```python
from build123d import *

# Parameters (mm, degrees)
F0_R     = 7.9375
F1_DEPTH = 14.2748
F2_R     = 1.1303
F3_DEPTH = 12.701


with BuildPart() as f1:
    # F0 (on Top) → F1 (new body)
    with BuildSketch(Plane.XY):
        Polygon((57.15, -9.525), (57.15, 9.525), (28.109774, 9.525), (28.109774, 3.175), (-28.109774, 3.175), (-28.109774, 9.525), (-95.25, 9.525), (-95.25, -9.525), align=None)
        with Locations((-44.45, 0)):
            Circle(F0_R, mode=Mode.SUBTRACT)
        with Locations((44.45, 0)):
            Circle(F0_R, mode=Mode.SUBTRACT)
    extrude(amount=F1_DEPTH)

    # F2 (on face) → F3 (cut, through all)
    with BuildSketch(Plane(origin=(0, 3.175, 0), x_dir=(-1, 0, 0), z_dir=(0, 1, 0))):
        with Locations((-17.907, 5.08)):
            Circle(F2_R)
        with Locations((17.907, 5.08)):
            Circle(F2_R)
    extrude(amount=-F3_DEPTH, mode=Mode.SUBTRACT)


solid = f1.part
```
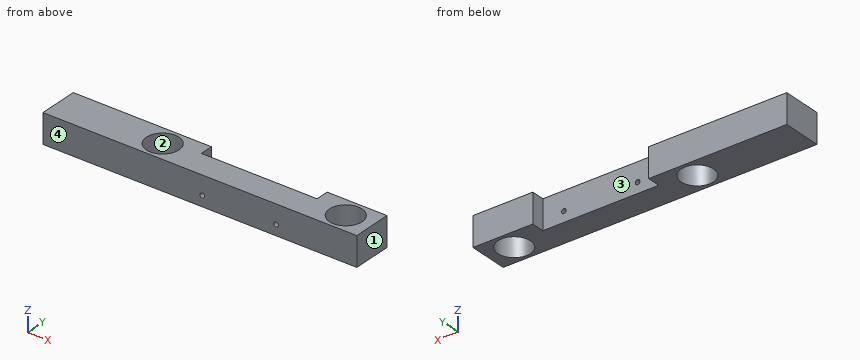
For this review, take the finished solid that the model builds, in its own axes (mm). Face numbers are marked on the shaded views. Coordinates: 2 decimals unless noted, no trailing zeros. Write each loop counter-clockwise with the first axis right and the second up, starting at its lowest first coordinate (ties: lowest second). Pieces come first, ordered by that corner, then holes. Notation, with made-up numbers: (-30.75, 82) -> (3.25, 82) arc R29 cw to (3.25, 110) -> close; hole circle Ø1 at (63.5, 16.25). An arc over 180 degrees is marked (long way). Put each result on its own line as item: value.
Q1. The part is to be moulded in two halves that separate along X. For the marked faces 1, 2, 3 and 4, say which applies: +X half, -X half, draft (parallel to the pull), parting line (faces both ways), or undercut.
From the geometry:
face 1: +X half
face 2: undercut
face 3: undercut
face 4: draft
Q2. Take a section at B-B, the plane z = 1.5. Count the separate pieces of the cut face and the enclosed holes in it, then the cut area to 3 significant figures.
From the geometry:
separate pieces: 1
enclosed holes: 2
area: 2,150 mm2
Q3. Take a section at A-A, the plane y = 0. State the section outline as (x, z) points, then the cut area to 3 significant figures.
From the geometry:
outline: (-95.25, 0) -> (-52.39, 0) -> (-52.39, 14.27) -> (-95.25, 14.27) -> close; (-36.51, 0) -> (36.51, 0) -> (36.51, 14.27) -> (-36.51, 14.27) -> close; (52.39, 0) -> (57.15, 0) -> (57.15, 14.27) -> (52.39, 14.27) -> close; hole circle Ø2.26 at (-17.91, 5.08); hole circle Ø2.26 at (17.91, 5.08)
area: 1,710 mm2
Q4. Take a section at D-D, the plane x = 43. State the section outline as (y, z) points (3 decimals).
From the geometry:
outline: (-9.525, 0) -> (-7.804, 0) -> (-7.804, 14.275) -> (-9.525, 14.275) -> close; (7.804, 0) -> (9.525, 0) -> (9.525, 14.275) -> (7.804, 14.275) -> close
Q5. Wall thickness on L1, parallel to X at y = -4.75, z = 1.25; L2, parallel to Y at x = -44.45, z = 9 (1 decimal); L3, parallel to X at y = -1, z = 13: over which ranges is each line inside the solid? List them lowest first.
From the geometry:
L1: x = -95.25 to -50.81, -38.09 to 38.09, 50.81 to 57.15
L2: y = -9.5 to -7.9, 7.9 to 9.5
L3: x = -95.25 to -52.32, -36.58 to 36.58, 52.32 to 57.15
Q6. Take a section at C-C, the plane x = -44.45. State the section outline as (y, z) points (1 decimal).
From the geometry:
outline: (-9.5, 0) -> (-7.9, 0) -> (-7.9, 14.3) -> (-9.5, 14.3) -> close; (7.9, 0) -> (9.5, 0) -> (9.5, 14.3) -> (7.9, 14.3) -> close
Q7. Clearance check with flat-ended pins moving along their axes: pin 1 Ø4 at (x, z) = (23.5, 2.5) entering from +Y (3 decimals); pin 2 Ø3.5 at (x, z) = (-17.907, 5.08) entering from -Y (3 decimals); pin 3 Ø1.8 at (x, z) = (17.907, 5.08) entering from -Y. State where each tip first meets the part, or that it passes through.
From the geometry:
pin 1: stops at y = 3.175
pin 2: stops at y = -9.525
pin 3: passes through
